Design review of the part built by this model. Coordinates are the model's own, in mm. Face numbers are marked on the shaded views. A direction names the side the tool comes from. Give positions to 0.01 mm unless a question says otherwise; leave off trailing zeros. Write each loop counter-clockwise with the first axis right and the second up, starting at its lowest first coordinate (ties: lowest second). Pieces come first, ordered by that corner, then holes. Notation, with made-up numbers: (47, 74.25) -> (75, 74.25) arc R24 cw to (75, 97.25) -> close; hole circle Ø9 at (45, 66.5). An arc over 180 degrees is marked (long way). Answer as a JSON object with one key per item and string values.
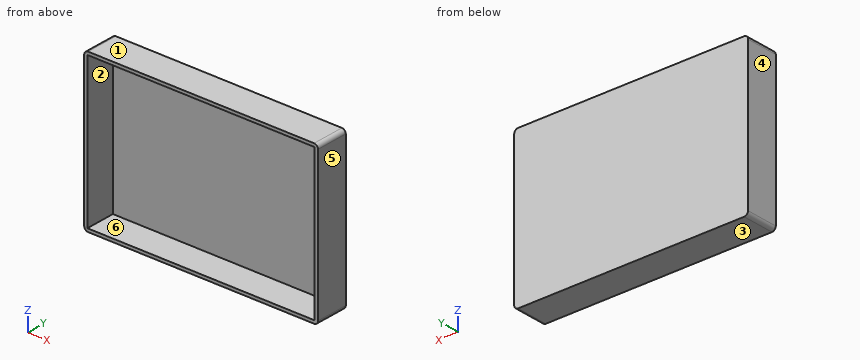
```python
from build123d import *

# Parameters (mm, degrees)
F1_DEPTH  = 25
F2_DEPTH  = 25
F3_DEPTH  = 25
F4_DEPTH  = 25
F5_DEPTH  = 25
F6_DEPTH  = 25
F7_DEPTH  = 25
F8_DEPTH  = 25
F0_W      = 87.680131197
F0_H      = 57.6011836529
F0_W_2    = 87.3793363571
F9_DEPTH  = 2
F10_DEPTH = 2
F11_DEPTH = 2
F12_DEPTH = 2
F13_R     = 3
F14_R     = 3
F15_R     = 3
F16_R     = 3


with BuildPart() as f1:
    # F0 (on Front) → F1 (new body)
    with BuildSketch(Plane.XZ):
        Polygon((0, 57.6011836529), (0, 60.0075013936), (-90.0864452124, 60.0075013936), (-87.680131197, 57.6011836529), align=None)
    extrude(amount=F1_DEPTH)

    # F0 (on Front) → F2 (join)
    with BuildSketch(Plane.XZ):
        Polygon((87.3793363571, 57.6011836529), (90.0864452124, 60.0075013936), (0, 60.0075013936), (0, 57.6011836529), align=None)
    extrude(amount=F2_DEPTH)

    # F0 (on Front) → F3 (join)
    with BuildSketch(Plane.XZ):
        Polygon((-87.680131197, 57.6011836529), (-90.0864452124, 60.0075013936), (-90.0864452124, 0), (-87.680131197, 0), align=None)
    extrude(amount=F3_DEPTH)

    # F0 (on Front) → F4 (join)
    with BuildSketch(Plane.XZ):
        Polygon((-87.680131197, 0), (-90.0864452124, 0), (-90.0864452124, -60.0075013936), (-87.680131197, -57.6011836529), align=None)
    extrude(amount=F4_DEPTH)

    # F0 (on Front) → F5 (join)
    with BuildSketch(Plane.XZ):
        Polygon((-90.0864452124, -60.0075013936), (-0.1503974199, -60.0075013936), (-0.1503974199, -57.6011836529), (-87.680131197, -57.6011836529), align=None)
    extrude(amount=F5_DEPTH)

    # F0 (on Front) → F6 (join)
    with BuildSketch(Plane.XZ):
        Polygon((-0.1503974199, -60.0075013936), (90.0864452124, -60.0075013936), (87.3793363571, -57.6011836529), (-0.1503974199, -57.6011836529), align=None)
    extrude(amount=F6_DEPTH)

    # F0 (on Front) → F7 (join)
    with BuildSketch(Plane.XZ):
        Polygon((90.0864452124, 0), (90.0864452124, 60.0075013936), (87.3793363571, 57.6011836529), (87.3793363571, 0), align=None)
    extrude(amount=F7_DEPTH)

    # F0 (on Front) → F8 (join)
    with BuildSketch(Plane.XZ):
        Polygon((90.0864452124, -60.0075013936), (90.0864452124, 0), (87.3793363571, 0), (87.3793363571, -57.6011836529), align=None)
    extrude(amount=F8_DEPTH)

    # F0 (on Front) → F9 (join)
    with BuildSketch(Plane.XZ):
        with Locations((-43.8400655985, 28.8005918264)):
            Rectangle(F0_W, F0_H)
        with Locations((43.6896681786, 28.8005918264)):
            Rectangle(F0_W_2, F0_H)
    extrude(amount=F9_DEPTH)

    # F0 (on Front) → F10 (join)
    with BuildSketch(Plane.XZ):
        with Locations((43.6896681786, 28.8005918264)):
            Rectangle(F0_W_2, F0_H)
    extrude(amount=F10_DEPTH)

    # F0 (on Front) → F11 (join)
    with BuildSketch(Plane.XZ):
        Polygon((-0.1503974199, -57.6011836529), (0, 0), (-87.680131197, 0), (-87.680131197, -57.6011836529), align=None)
    extrude(amount=F11_DEPTH)

    # F0 (on Front) → F12 (join)
    with BuildSketch(Plane.XZ):
        Polygon((87.3793363571, -57.6011836529), (87.3793363571, 0), (0, 0), (-0.1503974199, -57.6011836529), align=None)
    extrude(amount=F12_DEPTH)

    # F13
    f13_edges = [f1.edges().sort_by_distance(p)[0] for p in [
        (-90.086445, -12.5, 60.007501),
    ]]
    fillet(f13_edges, radius=F13_R)

    # F14
    f14_edges = [f1.edges().sort_by_distance(p)[0] for p in [
        (90.086445, -12.5, 60.007501),
    ]]
    fillet(f14_edges, radius=F14_R)

    # F15
    f15_edges = [f1.edges().sort_by_distance(p)[0] for p in [
        (90.086445, -12.5, -60.007501),
    ]]
    fillet(f15_edges, radius=F15_R)

    # F16
    f16_edges = [f1.edges().sort_by_distance(p)[0] for p in [
        (-90.086445, -12.5, -60.007501),
    ]]
    fillet(f16_edges, radius=F16_R)


solid = f1.part
```
(1) We need section B-B, the plane x = -74. State the section outline as (y, z) points.
Here are the results:
{"outline": "(-25, -60.01) -> (0, -60.01) -> (0, 60.01) -> (-25, 60.01) -> (-25, 57.6) -> (-2, 57.6) -> (-2, -57.6) -> (-25, -57.6) -> close"}
(2) The part is to be moulded in two halves that separate along Z. For the marked faces 1, 2, 3 and 4, say which applies: +Z half, -Z half, draft (parallel to the pull), parting line (faces both ways), or undercut.
Here are the results:
{"face 1": "+Z half", "face 2": "undercut", "face 3": "-Z half", "face 4": "draft"}
(3) Clearance check with a flat-ended pin moving along its axis: pin 1 (6 mm diameter, centred on x = 47, z = -19.5, fed in from -Y). State where the tip first meets the part, or that it passes through.
Here are the results:
{"pin 1": "stops at y = -2"}
(4) We need section A-A, the plane y = -13.5. State the section outline as (x, z) points, then the cut area to 3 significant figures.
Here are the results:
{"outline": "(-90.09, -57.01) arc R3 ccw to (-87.09, -60.01) -> (87.09, -60.01) arc R3 ccw to (90.09, -57.01) -> (90.09, 57.01) arc R3 ccw to (87.09, 60.01) -> (-87.09, 60.01) arc R3 ccw to (-90.09, 57.01) -> close; hole (-87.68, -57.6) -> (87.38, -57.6) -> (87.38, 57.6) -> (-87.68, 57.6) -> close", "area": "1,450 mm²"}
(5) For the marked faces 5 and 6, list the 3-axis set-ups (+Z, -Z, +X, -X, +Y, -Y) from which the entire face can be reached by the end or side of a thin tool; tool diameter is ignored.
Here are the results:
{"face 5": "+Z, -Z, +X, +Y, -Y", "face 6": "-Y"}
(6) For line 1 along Z through (x, y) = (76, -5.5); line 2 along X through (y, z) = (-2.25, 24.5); line 3 along Y through (x, z) = (76, 47), list the stretches that pass through material, from the lowest coordinate up.
Here are the results:
{"line 1": "z = -60.01 to -57.6, 57.6 to 60.01", "line 2": "x = -90.09 to -87.68, 87.38 to 90.09", "line 3": "y = -2 to 0"}
(7) We need section C-C, the plane z = -31. State the section outline as (x, y) points.
Here are the results:
{"outline": "(-90.09, -25) -> (-87.68, -25) -> (-87.68, -2) -> (87.38, -2) -> (87.38, -25) -> (90.09, -25) -> (90.09, 0) -> (-90.09, 0) -> close"}
